Source: CAD feature listing. Evaluate the final solid. Frame: model axes, mm. Coordinates: 2 decimals unless noted, no trailing zeros. Order: outer loops, then holes, each group sorted by start corner. A loop starts at its lowest first (then second) coordinate and runs counter-clockwise, first axis right, second up. Notation, with made-up numbers: (33.5, -16) -> (74.5, -16) arc R16 ccw to (74.5, -7) -> close; hole circle Ø11 at (-14, 71). An arc over 180 degrees is marked (long way). Write each question's results on one line, items separated by ' | '. Start each with the question number.
from build123d import *

# Parameters (mm, degrees)
SKETCH1_W           = 12.7
SKETCH1_H           = 10.922
BOSS_EXTRUDE1_DEPTH = 5.08
SKETCH2_R           = 0.7874
CUT_EXTRUDE1_DEPTH  = 5.08
FILLET1_R           = 2.54


with BuildPart() as part:
    # Sketch1 → Boss-Extrude1 (new body)
    with BuildSketch(Plane.XY):
        Rectangle(SKETCH1_W, SKETCH1_H)
    extrude(amount=BOSS_EXTRUDE1_DEPTH)

    # Sketch2 → Cut-Extrude1 (cut)
    with BuildSketch(Plane.XY):
        Circle(SKETCH2_R)
        with Locations((3.302, 0)):
            Circle(SKETCH2_R)
        with Locations((-3.302, 0)):
            Circle(SKETCH2_R)
    extrude(amount=CUT_EXTRUDE1_DEPTH, mode=Mode.SUBTRACT)

    # Fillet1
    fillet1_edges = [part.edges().sort_by_distance(p)[0] for p in [
        (-6.35, 5.461, 2.54),
        (6.35, 5.461, 2.54),
    ]]
    fillet(fillet1_edges, radius=FILLET1_R)


solid = part.part
(1) Section A-A on x = 0. Return the cut outline in (y, z).
(2) Line query: L1, parallel to Y at x = 0, z = 1.7; L2, parallel to X at y = -0.25, z = 3.3; L3, parallel to Y at x = 2.75, z = 1.8. Output: solid intervals per line, ascending.
(3) Draft query along X for faces 1 (the cylindrical face through (4.03, -0.3, 2.5)), 2 (the flat face through (0, -1, 5.08)), 3 (the cylindrical face through (-0.625, -0.479, 2.504)), 4 (the cylindrical face through (-5.626, 4.697, 2.576)). Return one class per face: released by +X, released by -X, zero draft, split by the parting line, or undercut.
(4) Section B-B on y = 0. Return the cut outline in (x, z), then the cut area to 3 significant figures.
(5) Section C-C on z = 2.25. Return the cut outline in (x, y), then the cut area to 3 significant figures.
(6) First-contact query: P1, Ø1.4, axis at x = 0, y = 0, coming from the -Z side. Flat tip, straight axial feed; report the tip coordinate or a pass-through.
(7) Section D-D on x = 5.25. Return the cut outline in (y, z), then the cut area to 3 significant figures.
Results list:
1) outline: (-5.46, 0) -> (-0.79, 0) -> (-0.79, 5.08) -> (-5.46, 5.08) -> close; (0.79, 0) -> (5.46, 0) -> (5.46, 5.08) -> (0.79, 5.08) -> close
2) L1: y = -5.46 to -0.79, 0.79 to 5.46 | L2: x = -6.35 to -4.05, -2.56 to -0.75, 0.75 to 2.56, 4.05 to 6.35 | L3: y = -5.46 to -0.56, 0.56 to 5.46
3) face 1: undercut | face 2: zero draft | face 3: undercut | face 4: released by -X
4) outline: (-6.35, 0) -> (-4.09, 0) -> (-4.09, 5.08) -> (-6.35, 5.08) -> close; (-2.51, 0) -> (-0.79, 0) -> (-0.79, 5.08) -> (-2.51, 5.08) -> close; (0.79, 0) -> (2.51, 0) -> (2.51, 5.08) -> (0.79, 5.08) -> close; (4.09, 0) -> (6.35, 0) -> (6.35, 5.08) -> (4.09, 5.08) -> close | area: 40.5 mm²
5) outline: (-6.35, -5.46) -> (6.35, -5.46) -> (6.35, 2.92) arc R2.54 ccw to (3.81, 5.46) -> (-3.81, 5.46) arc R2.54 ccw to (-6.35, 2.92) -> close; hole circle Ø1.57 at (-3.3, 0); hole circle Ø1.57 at (0, 0); hole circle Ø1.57 at (3.3, 0) | area: 130 mm²
6) P1: passes through
7) outline: (-5.46, 0) -> (5.01, 0) -> (5.01, 5.08) -> (-5.46, 5.08) -> close | area: 53.2 mm²
